Input: part model. Units: mm. Frame: model coordinates. A direction names the side the tool comes from. Round coordinates to 2 decimals unless told otherwise and drop trailing zeros. Loops run counter-clockwise (first coordinate to the right, second up) from the corner with the lowest first, then second, coordinate; pieces in that order, holes last. Notation, with made-up numbers: M 29.25,66 L 63.25,66 A9 ccw 63.25,77 Z; hole C 39,89.5 d10. An arc over 180 degrees is marked long. Return JSON: item names as keys, results as strings. Group by question number.
1) Contact query for flat-ended pins moving along their axis: P1, Ø1, axis at x = 53, y = 2.5, coming from the +Z side; P2, Ø1.6, axis at x = 46.5, y = 1, coming from the +Z side. Output: stop coordinate, or through.
2) Section A-A (z = 8). Output: boundary loops of the cut face in (x, y) (3 decimals), plus the area to 3 significant figures.
3) Section C-C (x = 7.5). Output: boundary loops of the cut face in (y, z) (3 decimals).
4) Section B-B (z = 10.75). Count the separate pieces of the cut face and the enclosed holes in it, plus the area to 3 significant figures.
5) Section D-D (x = 46.5). Output: boundary loops of the cut face in (y, z) (3 decimals).
6) Material intervals for line 1 (X direction, y = 0.8, z = 9) (3 decimals); line 2 (Z direction, x = 13, y = 2.75); line 3 (Z direction, x = 22.5, y = 2.45), sorted ascending. Write a range as from..to.
7) Access query for faces 4 (the face through (33, 2, 12.7)), 5 (the face through (19.225, 2, 11)). Directions: +Z, -Z, +X, -X, +Y, -Y. A direction counts if a zero-diameter tool reaches every point of the face in a straight line with its end or side. Return the directions, or none.
8) Mould query, pull axis X, two halves, no side actions, for faces 1 (the face through (38, 3.175, 5)), 2 (the face through (0, 2, 6)), 3 (the face through (70, 2, 9.7)). Classes: +X half, -X half, draft (parallel to the pull), parting line (faces both ways), or undercut.
from build123d import *

# Parameters (mm, degrees)
SKETCH1_W           = 76.2
SKETCH1_H           = 12.7
BOSS_EXTRUDE1_DEPTH = 3.175
SKETCH4_W           = 3.175
SKETCH4_H           = 6.35
CUT_EXTRUDE1_DEPTH  = 4.175
LPATTERN1_COUNT     = 4
LPATTERN1_PITCH     = 15.875
CUT_EXTRUDE2_DEPTH  = 4.175
LPATTERN2_COUNT     = 5
LPATTERN2_PITCH     = 15.875


with BuildPart() as part:
    # Sketch1 → Boss-Extrude1 (new body)
    with BuildSketch(Plane(origin=(0, 0, 0), x_dir=(1, 0, 0), z_dir=(0, 1, 0))):
        with Locations((38.1, -6.35)):
            Rectangle(SKETCH1_W, SKETCH1_H)
    extrude(amount=BOSS_EXTRUDE1_DEPTH)

    # Sketch4 → Cut-Extrude1 (cut, through all)
    with BuildSketch(Plane(origin=(0, 3.175, 0), x_dir=(1, 0, 0), z_dir=(0, 1, 0))):
        with Locations((14.2875, -9.525)):
            Rectangle(SKETCH4_W, SKETCH4_H)
    cut_extrude1 = extrude(amount=-CUT_EXTRUDE1_DEPTH, mode=Mode.SUBTRACT)

    # LPattern1: Cut-Extrude1 ×4
    with Locations(*[(i * LPATTERN1_PITCH, 0, 0) for i in range(1, LPATTERN1_COUNT)]):
        add(cut_extrude1, mode=Mode.SUBTRACT)

    # Sketch5 → Cut-Extrude2 (cut, through all)
    with BuildSketch(Plane(origin=(0, 3.175, 0), x_dir=(1, 0, 0), z_dir=(0, 1, 0))):
        Polygon((6.35, -9.7), (9.35, -9.7), (9.35, -12.7), (3.35, -12.7), (3.35, -9.7), align=None)
    cut_extrude2 = extrude(amount=-CUT_EXTRUDE2_DEPTH, mode=Mode.SUBTRACT)

    # LPattern2: Cut-Extrude2 ×5
    with Locations(*[(i * LPATTERN2_PITCH, 0, 0) for i in range(1, LPATTERN2_COUNT)]):
        add(cut_extrude2, mode=Mode.SUBTRACT)


solid = part.part
Returned:
{
 "1": {"P1": "stops at z = 9.7", "P2": "stops at z = 6.35"},
 "2": {"outline": "M 0,0 L 12.7,0 L 12.7,3.175 L 0,3.175 Z; M 15.875,0 L 28.575,0 L 28.575,3.175 L 15.875,3.175 Z; M 31.75,0 L 44.45,0 L 44.45,3.175 L 31.75,3.175 Z; M 47.625,0 L 60.325,0 L 60.325,3.175 L 47.625,3.175 Z; M 63.5,0 L 76.2,0 L 76.2,3.175 L 63.5,3.175 Z", "area": "202 mm^2"},
 "3": {"outline": "M 0,0 L 3.175,0 L 3.175,9.7 L 0,9.7 Z"},
 "4": {"separate pieces": "10", "enclosed holes": "0", "area": "106 mm^2"},
 "5": {"outline": "M 0,0 L 3.175,0 L 3.175,6.35 L 0,6.35 Z"},
 "6": {"line 1": "x = 0..12.7, 15.875..28.575, 31.75..44.45, 47.625..60.325, 63.5..76.2", "line 2": "z = 0..6.35", "line 3": "z = 0..9.7"},
 "7": {"face 4": "+Z, +X, -X, +Y, -Y", "face 5": "+Z, +Y, -Y"},
 "8": {"face 1": "draft", "face 2": "-X half", "face 3": "undercut"}
}
